The model under review builds one solid part; all positions refer to its coordinate system, in mm. A direction names the side the tool comes from. Round coordinates to 2 decimals unless told otherwise and drop trailing zeros. Loops run counter-clockwise (first coordinate to the right, second up) from the corner with the lowest first, then second, coordinate; pieces in that order, holes last. Notation, with made-up numbers: M 69.5,73 L 113.5,73 A17 ccw 113.5,93 Z; hole C 78,86 d7. An arc over 180 degrees is marked long. Use a Markdown table: item, result. Add a question column.
```python
from build123d import *

# Parameters (mm, degrees)
SKETCH_1_W                   = 50
SKETCH_1_H                   = 27.3
EXTRUDE_1_DEPTH              = 22
SKETCH_2_W                   = 30
SKETCH_2_H                   = 30
EXTRUDE_2_DEPTH              = 28
SKETCH_3_R                   = 6
CUT_EXTRUDE_1_DEPTH          = 68.411052506
CHAMFER_1_SIZE               = 3
CHAMFER_2_SIZE               = 1
HOLE_WIZARD_M4_1_D           = 4.5
HOLE_WIZARD_M4_1_CBORE_D     = 8
HOLE_WIZARD_M4_1_CBORE_DEPTH = 4


with BuildPart() as part:
    # 스케치1 → 보스-돌출1 (new body)
    with BuildSketch(Plane.XY):
        with Locations((25, 13.65)):
            Rectangle(SKETCH_1_W, SKETCH_1_H)
    extrude(amount=EXTRUDE_1_DEPTH)

    # 스케치2 → 보스-돌출2 (add)
    with BuildSketch(Plane.XY.offset(22)):
        with Locations((25, 20.5)):
            Rectangle(SKETCH_2_W, SKETCH_2_H)
    extrude(amount=-EXTRUDE_2_DEPTH)

    # 스케치3 → 컷-돌출1 (cut, through all)
    with BuildSketch(Plane(origin=(0, 0, -6), x_dir=(-1, 0, 0), z_dir=(0, 0, -1))):
        with Locations((-25, 20)):
            Circle(SKETCH_3_R)
    extrude(amount=-CUT_EXTRUDE_1_DEPTH, mode=Mode.SUBTRACT)

    # 모따기1
    chamfer_1_edges = [part.edges().sort_by_distance(p)[0] for p in [
        (40, 35.5, 8),
        (10, 35.5, 8),
    ]]
    chamfer(chamfer_1_edges, length=CHAMFER_1_SIZE)

    # 모따기2
    chamfer_2_edges = [part.edges().sort_by_distance(p)[0] for p in [
        (0, 27.3, 11),
        (50, 27.3, 11),
    ]]
    chamfer(chamfer_2_edges, length=CHAMFER_2_SIZE)

    # M4 소켓 머리 캡 나사용 카운터보어1 (through all)
    with Locations(Plane(origin=(0, 27.3, 0), x_dir=(1, 0, 0), z_dir=(0, 1, 0))):
        with Locations((44, -5), (44, -17), (6, -17), (6, -5)):
            CounterBoreHole(HOLE_WIZARD_M4_1_D / 2, HOLE_WIZARD_M4_1_CBORE_D / 2, HOLE_WIZARD_M4_1_CBORE_DEPTH)


solid = part.part
```
(1) To check wall thickness, follow probe 1 along Z at (x, y) = (44, 25.5); probe 2 along Y at (x, z) = (25, 9.5); probe 3 along Z at (x, y) = (6.5, 4.5). State the ranges of each line that lie inside material, in increasing order.
(2) Consider section C-C, the plane x = 25. Give the boundary of the cut face in (y, z), then the cut area to 3 significant figures.
(3) For faces 1 (the face through (25, 5.5, -3)), 2 (the face through (29.76, 16.35, 7.8)), 3 (the face through (8, 23.3, 7)), 4 (the face through (45.786, 11.487, 18.369)), 5 (the face through (4, 27.3, 11)), list the 3-axis set-ups (+Z, -Z, +X, -X, +Y, -Y) from which the entire face can be reached by the end or side of a thin tool; tool diameter is ignored.
(4) Insertion check: pin 1 Ø3 at (x, z) = (42.5, 15.5) entering from +Y; pin 2 Ø5 at (x, z) = (44, 5) entering from -Y; pin 3 Ø1.5 at (x, y) = (8, 21.5) entering from -Z; pin 4 Ø6.5 at (x, z) = (42.5, 18) entering from +Y. Each pin has a flat end and moves straight along its axis. Give the tip position at first contact, or say it passes through.
(5) Consider section B-B, the plane y = 20. Give the boundary of the cut face in (x, z).
(6) Consider section A-A, the plane x = 6. Give the boundary of the cut face in (y, z).
(7) Consider section D-D, the plane y = 25. Give the boundary of the cut face in (x, z).
(8) Draft analysis for pull direction Z (two halves, no side actions). For faces 6 (the face through (25, 0, 11)), 7 (the face through (5.133, 25.328, 8.905)), 8 (the face through (31.5, 20.7, -6)), state which applies: released by +Z, released by -Z, zero draft, split by the parting line, or undercut.
Found:
| question | item | result |
|---|---|---|
| 1 | probe 1 | z = 0 to 1, 9 to 13, 21 to 22 |
| 1 | probe 2 | y = 0 to 14, 26 to 35.5 |
| 1 | probe 3 | z = 0 to 2.81, 7.19 to 14.81, 19.19 to 22 |
| 2 | outline | M 0,0 L 5.5,0 L 5.5,-6 L 14,-6 L 14,22 L 0,22 Z; M 26,-6 L 35.5,-6 L 35.5,22 L 26,22 Z |
| 2 | area | 625 mm^2 |
| 3 | face 1 | -Z, +X, -X, -Y |
| 3 | face 2 | +Z, -Z |
| 3 | face 3 | +Y |
| 3 | face 4 | +Y, -Y |
| 3 | face 5 | +Z, -Z, -X, +Y |
| 4 | pin 1 | stops at y = 23.3 |
| 4 | pin 2 | stops at y = 0 |
| 4 | pin 3 | stops at z = 0 |
| 4 | pin 4 | stops at y = 33.25 |
| 5 | outline | M 0,0 L 10,0 L 10,-6 L 19,-6 L 19,22 L 0,22 Z; M 31,-6 L 40,-6 L 40,0 L 50,0 L 50,22 L 31,22 Z; hole C 6,5 d4.5; hole C 6,17 d4.5; hole C 44,5 d4.5; hole C 44,17 d4.5 |
| 6 | outline | M 0,0 L 27.3,0 L 27.3,1 L 23.3,1 L 23.3,2.75 L 0,2.75 Z; M 0,7.25 L 23.3,7.25 L 23.3,9 L 27.3,9 L 27.3,13 L 23.3,13 L 23.3,14.75 L 0,14.75 Z; M 0,19.25 L 23.3,19.25 L 23.3,21 L 27.3,21 L 27.3,22 L 0,22 Z |
| 7 | outline | M 0,0 L 10,0 L 10,-6 L 21.68,-6 L 21.68,22 L 0,22 Z; M 28.32,-6 L 40,-6 L 40,0 L 50,0 L 50,22 L 28.32,22 Z; hole C 6,5 d8; hole C 6,17 d8; hole C 44,5 d8; hole C 44,17 d8 |
| 8 | face 6 | zero draft |
| 8 | face 7 | undercut |
| 8 | face 8 | released by -Z |
